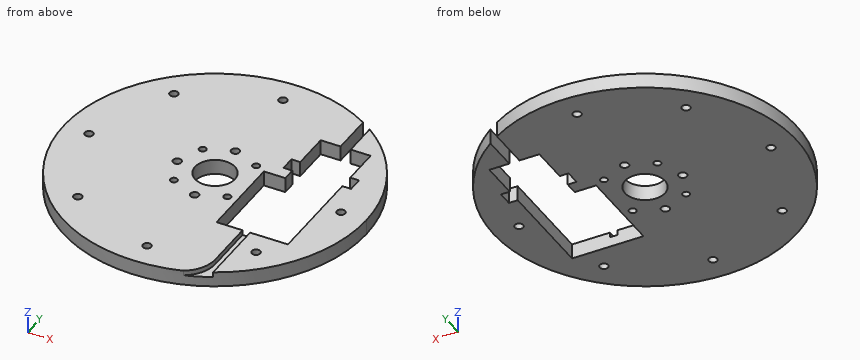
```python
from build123d import *
from build123d.topology import SkipClean

# Parameters (mm, degrees)
SKETCH1_R           = 60
SKETCH1_R_2         = 8
SKETCH1_R_3         = 1.75
SKETCH1_R_4         = 1.5
BOSS_EXTRUDE1_DEPTH = 6
CUT_EXTRUDE1_DEPTH  = 86.064681273
MOVE_FACE1_BY       = 0.08
MOVE_FACE1_2_BY     = 0.08
MOVE_FACE1_3_BY     = 0.08
MOVE_FACE1_4_BY     = 0.08
MOVE_FACE1_5_BY     = 0.08
MOVE_FACE1_6_BY     = 0.08
MOVE_FACE1_7_BY     = 0.08
MOVE_FACE1_8_BY     = 0.08
MOVE_FACE1_9_BY     = 0.08
MOVE_FACE1_10_BY    = 0.08
MOVE_FACE1_11_BY    = 0.08
MOVE_FACE1_12_BY    = 0.08
MOVE_FACE1_13_BY    = 0.08
MOVE_FACE1_14_BY    = 0.08
MOVE_FACE1_15_BY    = 0.08
MOVE_FACE1_16_BY    = 0.08
MOVE_FACE1_17_BY    = 0.08
MOVE_FACE1_18_BY    = 0.08
MOVE_FACE1_19_BY    = 0.08
MOVE_FACE1_20_BY    = 0.08
MOVE_FACE1_21_BY    = 0.08
MOVE_FACE1_22_BY    = 0.08
MOVE_FACE1_23_BY    = 0.08
MOVE_FACE1_24_BY    = 0.08
MOVE_FACE1_25_BY    = 0.08
MOVE_FACE1_26_BY    = 0.08
MOVE_FACE1_27_BY    = 0.08
MOVE_FACE1_28_BY    = 0.08
MOVE_FACE1_29_BY    = 0.08
MOVE_FACE1_30_BY    = 0.08
CUT_EXTRUDE2_DEPTH  = 2
SKETCH4_W           = 4
SKETCH4_H           = 40
CUT_EXTRUDE3_DEPTH  = 86.177536945


with BuildPart() as part:
    # Sketch1 → Boss-Extrude1 (new body)
    with BuildSketch(Plane.XY):
        Circle(SKETCH1_R)
        Circle(SKETCH1_R_2, mode=Mode.SUBTRACT)
        with Locations((0, -15)):
            Circle(SKETCH1_R_3, mode=Mode.SUBTRACT)
        with Locations((10.606601718, -10.606601718)):
            Circle(SKETCH1_R_4, mode=Mode.SUBTRACT)
        with Locations((0, -50)):
            Circle(SKETCH1_R_3, mode=Mode.SUBTRACT)
        with Locations((-15, 0)):
            Circle(SKETCH1_R_3, mode=Mode.SUBTRACT)
        with Locations((-10.606601718, -10.606601718)):
            Circle(SKETCH1_R_4, mode=Mode.SUBTRACT)
        with Locations((0, 15)):
            Circle(SKETCH1_R_3, mode=Mode.SUBTRACT)
        with Locations((-10.606601718, 10.606601718)):
            Circle(SKETCH1_R_4, mode=Mode.SUBTRACT)
        with Locations((10.606601718, 10.606601718)):
            Circle(SKETCH1_R_4, mode=Mode.SUBTRACT)
        with Locations((-35.355339059, -35.355339059)):
            Circle(SKETCH1_R_3, mode=Mode.SUBTRACT)
        with Locations((-50, 0)):
            Circle(SKETCH1_R_3, mode=Mode.SUBTRACT)
        with Locations((-35.355339059, 35.355339059)):
            Circle(SKETCH1_R_3, mode=Mode.SUBTRACT)
        with Locations((0, 50)):
            Circle(SKETCH1_R_3, mode=Mode.SUBTRACT)
        with Locations((50, 0)):
            Circle(SKETCH1_R_3, mode=Mode.SUBTRACT)
        with Locations((35.355339059, -35.355339059)):
            Circle(SKETCH1_R_3, mode=Mode.SUBTRACT)
    extrude(amount=BOSS_EXTRUDE1_DEPTH)

    # Sketch2 → Cut-Extrude1 (cut, through all)
    with BuildSketch(Plane.XY.offset(6)):
        Polygon((14.5, -26), (43, -26), (43, 14), (46.5, 14), (46.5, 20), (43, 20), (43, 35), (23, 35), (23, 20), (19.5, 20), (19.5, 14), (23, 14), (23, 9), (14.5, 9), align=None)
    extrude(amount=-CUT_EXTRUDE1_DEPTH, mode=Mode.SUBTRACT)

    # Move Face1: a curved face moved outward by 0.08
    add(Solid.thicken(part.faces().sort_by_distance((-60, 0, 3))[0], MOVE_FACE1_BY))

    # Move Face1 2: a face moved outward by 0.08
    extrude(part.faces().sort_by_distance((23, 11.5, 3))[0], amount=MOVE_FACE1_2_BY, dir=(1, 0, 0))

    # Move Face1 3: a curved face moved outward by 0.08
    add(Solid.thicken(part.faces().sort_by_distance((-8, 0, 3))[0], MOVE_FACE1_3_BY))

    # Move Face1 4: a curved face moved outward by 0.08
    add(Solid.thicken(part.faces().sort_by_distance((-1.75, -15, 3))[0], MOVE_FACE1_4_BY))

    # Move Face1 5: a curved face moved outward by 0.08
    add(Solid.thicken(part.faces().sort_by_distance((9.106601718, -10.606601718, 3))[0], MOVE_FACE1_5_BY))

    # Move Face1 6: a curved face moved outward by 0.08
    add(Solid.thicken(part.faces().sort_by_distance((-1.75, -50, 3))[0], MOVE_FACE1_6_BY))

    # Move Face1 7: a curved face moved outward by 0.08
    add(Solid.thicken(part.faces().sort_by_distance((-16.75, 0, 3))[0], MOVE_FACE1_7_BY))

    # Move Face1 8: a curved face moved outward by 0.08
    add(Solid.thicken(part.faces().sort_by_distance((-12.106601718, -10.606601718, 3))[0], MOVE_FACE1_8_BY))

    # Move Face1 9: a curved face moved outward by 0.08
    add(Solid.thicken(part.faces().sort_by_distance((-1.75, 15, 3))[0], MOVE_FACE1_9_BY))

    # Move Face1 10: a curved face moved outward by 0.08
    add(Solid.thicken(part.faces().sort_by_distance((-12.106601718, 10.606601718, 3))[0], MOVE_FACE1_10_BY))

    # Move Face1 11: a curved face moved outward by 0.08
    add(Solid.thicken(part.faces().sort_by_distance((9.106601718, 10.606601718, 3))[0], MOVE_FACE1_11_BY))

    # Move Face1 12: a curved face moved outward by 0.08
    add(Solid.thicken(part.faces().sort_by_distance((-37.105339059, -35.355339059, 3))[0], MOVE_FACE1_12_BY))

    # Move Face1 13: a curved face moved outward by 0.08
    add(Solid.thicken(part.faces().sort_by_distance((-51.75, 0, 3))[0], MOVE_FACE1_13_BY))

    # Move Face1 14: a curved face moved outward by 0.08
    add(Solid.thicken(part.faces().sort_by_distance((-37.105339059, 35.355339059, 3))[0], MOVE_FACE1_14_BY))

    # Move Face1 15: a curved face moved outward by 0.08
    add(Solid.thicken(part.faces().sort_by_distance((-1.75, 50, 3))[0], MOVE_FACE1_15_BY))

    # Move Face1 16: a curved face moved outward by 0.08
    add(Solid.thicken(part.faces().sort_by_distance((48.25, 0, 3))[0], MOVE_FACE1_16_BY))

    # Move Face1 17: a curved face moved outward by 0.08
    add(Solid.thicken(part.faces().sort_by_distance((33.605339059, -35.355339059, 3))[0], MOVE_FACE1_17_BY))

    # Move Face1 18: a face moved outward by 0.08
    extrude(part.faces().sort_by_distance((23, 27.5, 3))[0], amount=MOVE_FACE1_18_BY, dir=(1, 0, 0))

    # Move Face1 19: a face moved outward by 0.08
    extrude(part.faces().sort_by_distance((18.75, 9, 3))[0], amount=MOVE_FACE1_19_BY, dir=(0, -1, 0))

    # Move Face1 20: a face moved outward by 0.08
    extrude(part.faces().sort_by_distance((21.25, 14, 3))[0], amount=MOVE_FACE1_20_BY, dir=(0, 1, 0))

    # Move Face1 21: a face moved outward by 0.08
    extrude(part.faces().sort_by_distance((21.25, 20, 3))[0], amount=MOVE_FACE1_21_BY, dir=(0, -1, 0))

    # Move Face1 22: a face moved outward by 0.08
    extrude(part.faces().sort_by_distance((33, 35, 3))[0], amount=MOVE_FACE1_22_BY, dir=(0, -1, 0))

    # Move Face1 23: a face moved outward by 0.08
    extrude(part.faces().sort_by_distance((28.75, -26, 3))[0], amount=MOVE_FACE1_23_BY, dir=(0, 1, 0))

    # Move Face1 24: a face moved outward by 0.08
    extrude(part.faces().sort_by_distance((43, -6, 3))[0], amount=MOVE_FACE1_24_BY, dir=(-1, 0, 0))

    # Move Face1 25: a face moved outward by 0.08
    extrude(part.faces().sort_by_distance((44.75, 14, 3))[0], amount=MOVE_FACE1_25_BY, dir=(0, 1, 0))

    # Move Face1 26: a face moved outward by 0.08
    extrude(part.faces().sort_by_distance((46.5, 17, 3))[0], amount=MOVE_FACE1_26_BY, dir=(-1, 0, 0))

    # Move Face1 27: a face moved outward by 0.08
    extrude(part.faces().sort_by_distance((44.75, 20, 3))[0], amount=MOVE_FACE1_27_BY, dir=(0, -1, 0))

    # Move Face1 28: a face moved outward by 0.08
    extrude(part.faces().sort_by_distance((43, 27.5, 3))[0], amount=MOVE_FACE1_28_BY, dir=(-1, 0, 0))

    # Move Face1 29: a face moved outward by 0.08
    extrude(part.faces().sort_by_distance((19.5, 17, 3))[0], amount=MOVE_FACE1_29_BY, dir=(1, 0, 0))

    # Move Face1 30: a face moved outward by 0.08
    extrude(part.faces().sort_by_distance((14.5, -8.5, 3))[0], amount=MOVE_FACE1_30_BY, dir=(1, 0, 0))

    # Sketch3 → Cut-Extrude2 (cut)
    with BuildSketch(Plane.XY.offset(6)):
        with BuildLine():
            Line((24.91040122, -45.959), (24.91040122, -25.92))
            Line((24.91040122, -25.92), (27.91040122, -25.92))
            Line((27.91040122, -25.92), (27.91040122, -58.86940122))
            Line((27.91040122, -58.86940122), (12, -58.86940122))
            ThreePointArc((12, -58.86940122), (21.12903225, -55.08803225), (24.91040122, -45.959))
        make_face()
    extrude(amount=-CUT_EXTRUDE2_DEPTH, mode=Mode.SUBTRACT)

    # Sketch4 → Cut-Extrude3 (cut, through all)
    with SkipClean():  # the faces are left unmerged after this step: merging them gives an invalid solid
        with BuildSketch(Plane.XY.offset(6)):
            with Locations((33, 34.92)):
                Rectangle(SKETCH4_W, SKETCH4_H)
        extrude(amount=-CUT_EXTRUDE3_DEPTH, mode=Mode.SUBTRACT)


solid = part.part
```
CAD build for the part. Positions are in the model's coordinates, mm. Coordinates: 2 decimals unless noted, no trailing zeros. Loops run counter-clockwise (first coordinate to the right, second up) from the corner with the lowest first, then second, coordinate; pieces in that order, holes last. Notation, with made-up numbers: (54.25, -11.75) - (85.25, -11.75) arc R31 cw to (85.25, 21.25) - close; hole circle Ø8 at (-11, -30.75). An arc over 180 degrees is marked (long way). Use CSV: the item, a comma, the result in double quotes. Start each with the question number.
Q1. Cut at C-C, the plane y = -15. List the corners of the cut face in (x, z), then the cut area to 3 significant figures.
Q2. Probe probe 1 along Y at (x, z) = (0, 4.15); probe 2 along Y at (x, z) = (-35, 4.65); probe 3 along X at (y, z) = (35, 3.6). List the from-to ranges inside material, lowest first. Write a range as from..to.
Q3. Cut at A-A, the plane x = 0. List the corners of the cut face in (y, z), then the cut area to 3 significant figures.
Q4. Cut at B-B, the plane y = -50. List the corners of the cut face in (x, z).
Q5. Drop flat-ended pins along their axis: P1, Ø1, axis at y = 18.5, z = 4.5, coming from the -X side; P2, Ø2, axis at y = -33.5, z = 5.5, coming from the -X side; P3, Ø1.6, axis at y = -32.5, z = 5.5, coming from the +X side. Give the stop position or say it passes through.
Q6. Cut at D-D, the plane x = -50. List the corners of the cut face in (y, z).
Here are the results:
1,outline,"(-58.18, 0) - (-1.67, 0) - (-1.67, 6) - (-58.18, 6) - close; (1.67, 0) - (14.58, 0) - (14.58, 6) - (1.67, 6) - close; (42.92, 0) - (58.18, 0) - (58.18, 6) - (42.92, 6) - close"
1,area,"508 mm2"
2,probe 1,"-60.08..-51.67, -48.33..-16.67, -13.33..-7.92, 7.92..13.33, 16.67..48.33, 51.67..60.08"
2,probe 2,"-48.83..-36.99, -33.72..33.72, 36.99..48.83"
2,probe 3,"-48.83..-36.99, -33.72..31, 35..48.83"
3,outline,"(-60.08, 0) - (-51.67, 0) - (-51.67, 6) - (-60.08, 6) - close; (-48.33, 0) - (-16.67, 0) - (-16.67, 6) - (-48.33, 6) - close; (-13.33, 0) - (-7.92, 0) - (-7.92, 6) - (-13.33, 6) - close; (7.92, 0) - (13.33, 0) - (13.33, 6) - (7.92, 6) - close; (16.67, 0) - (48.33, 0) - (48.33, 6) - (16.67, 6) - close; (51.67, 0) - (60.08, 0) - (60.08, 6) - (51.67, 6) - close"
3,area,"546 mm2"
4,outline,"(-33.31, 0) - (-1.67, 0) - (-1.67, 6) - (-33.31, 6) - close; (1.67, 0) - (33.31, 0) - (33.31, 6) - (27.91, 6) - (27.91, 4) - (24.26, 4) - (24.26, 6) - (1.67, 6) - close"
5,P1,"x = -57.32"
5,P2,"x = -50.53"
5,P3,"x = 51.04"
6,outline,"(-33.31, 0) - (-1.67, 0) - (-1.67, 6) - (-33.31, 6) - close; (1.67, 0) - (33.31, 0) - (33.31, 6) - (1.67, 6) - close"
